Check sheet for the modelled part. Datum: model origin and axes. Units: mm. Face numbers are marked on the shaded views. A direction names the side the tool comes from. Give positions to 0.01 mm unless a question says otherwise; leave off trailing zeros. Loops run counter-clockwise (first coordinate to the right, second up) from the corner with the lowest first, then second, coordinate; pieces in that order, holes last. Notation, with made-up numbers: M -5.75,25.5 L 53.25,25.5 A7 cw 53.25,37.5 Z; hole C 13,-13.5 d4. An arc over 180 degrees is marked long. Use one line per item in the form item = value.
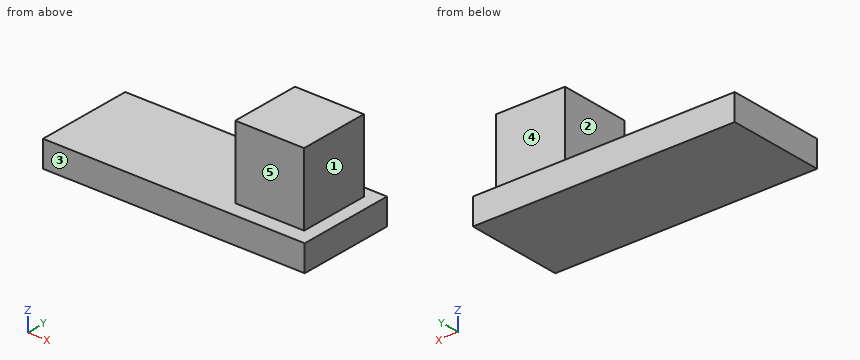
from build123d import *

# Parameters (mm, degrees)
F0_W     = 200
F0_H     = 20
F1_DEPTH = 75
F2_W     = 52.6148378849
F2_H     = 54.3804401532
F3_DEPTH = 55


# Not quite as in the source:
# - a feature names something its author has since deleted; it is built from what else it names


with BuildPart() as f1:
    # F0 (on Front) → F1 (new body)
    with BuildSketch(Plane.XZ):
        with Locations((39.6226420999, -12.8532575865)):
            Rectangle(F0_W, F0_H)
    extrude(amount=F1_DEPTH)

    # F2 (on face) → F3 (join)
    with BuildSketch(Plane.XY.offset(-2.8532575865)):
        with Locations((103.0974239111, -36.1731755547)):
            Rectangle(F2_W, F2_H)
    extrude(amount=F3_DEPTH)


solid = f1.part
1) Section check A-A (y = -29). Record the cut outline in (x, z), then the cut area to 3 significant figures.
Evaluation:
outline = M -60.38,-22.85 L 139.62,-22.85 L 139.62,-2.85 L 129.4,-2.85 L 129.4,52.15 L 76.79,52.15 L 76.79,-2.85 L -60.38,-2.85 Z
area = 6,890 mm^2
2) Section check D-D (x = 70). Record the cut outline in (y, z).
Evaluation:
outline = M -75,-22.85 L 0,-22.85 L 0,-2.85 L -75,-2.85 Z
3) Section check B-B (x = 107.5). Record the cut outline in (y, z), then the cut area to 3 significant figures.
Evaluation:
outline = M -75,-22.85 L 0,-22.85 L 0,-2.85 L -8.98,-2.85 L -8.98,52.15 L -63.36,52.15 L -63.36,-2.85 L -75,-2.85 Z
area = 4,490 mm^2
4) Section check C-C (z = 10). Record the cut outline in (x, y), then the cut area to 3 significant figures.
Evaluation:
outline = M 76.79,-63.36 L 129.4,-63.36 L 129.4,-8.98 L 76.79,-8.98 Z
area = 2,860 mm^2
5) Scan lines: line 1 (X direction, y = -36, z = 12); line 2 (Z direction, x = -27, y = -25); line 3 (Y direction, x = 122.5, z = 34). Record each from-to range of solid material in increasing order.
Evaluation:
line_1 = 76.79 to 129.4
line_2 = -22.85 to -2.85
line_3 = -63.36 to -8.98
6) Set-up check for the marked faces 1, 2, 3, 4 and 5: record each of +Z, -Z, +X, -X, +Y, -Y from which the full face is reachable in a straight line by a thin tool's end or side.
Evaluation:
face_1 = +Z, +X, +Y, -Y
face_2 = +Z, -X, +Y, -Y
face_3 = +Z, -Z, +X, -X, -Y
face_4 = +Z, +X, -X, +Y
face_5 = +Z, +X, -X, -Y
7) Depth check by flat-ended pin: pin 1 Ø10 at (y, z) = (-40, 34) entering from -X; pin 2 Ø10 at (x, y) = (-10, -44) entering from +Z; pin 3 Ø4 at (x, z) = (104.5, 0.5) entering from +Y. Enter the tip coordinate at first touch or a pass-through.
Evaluation:
pin_1 = 76.79
pin_2 = -2.85
pin_3 = -8.98
